```python
from build123d import *

# Parameters (mm, degrees)
CYLINDER004_R             = 1.65
CYLINDER004_DEPTH         = 15
CYLINDER004_ROLL_ANGLE    = -90
PAD004_DEPTH              = 2.5
FUSION006_PLACEMENT_ANGLE = 90
CYLINDER005_R             = 1.65
CYLINDER005_DEPTH         = 15
CYLINDER005_ROLL_ANGLE    = -90
PAD002_DEPTH              = 2.5
FUSION005_PLACEMENT_ANGLE = 90
PAD003_DEPTH              = 3
BOX009_W                  = 4
BOX009_H                  = 4
BOX009_DEPTH              = 10
BOX011_W                  = 24
BOX011_H                  = 12
BOX011_DEPTH              = 10
BOX010_W                  = 34
BOX010_H                  = 27
BOX010_DEPTH              = 3
FUSION007_PLACEMENT_ANGLE = -90


with BuildPart() as cylinder004:
    # Cylinder004 → Cylinder004 (new body)
    with BuildSketch(Plane.XY):
        Circle(CYLINDER004_R)
    extrude(amount=CYLINDER004_DEPTH)


with BuildPart() as cylinder004_1:
    # Cylinder004 roll: moved
    add(cylinder004.part.rotate(Axis((0, 0, 0), (1, 0, 0)), CYLINDER004_ROLL_ANGLE))


with BuildPart() as cylinder004_2:
    # Cylinder004 placement: moved
    add(cylinder004_1.part)


with BuildPart() as obj1:
    # Sketch → Pad004 (new body)
    with BuildSketch(Plane.XZ):
        Polygon((-3.348631, 0), (-1.674316, 2.9), (1.674316, 2.9), (3.348631, 0), (1.674316, -2.9), (-1.674316, -2.9), align=None)
    extrude(amount=PAD004_DEPTH)

    # Fusion006: union Cylinder004
    add(cylinder004_2.part)


with BuildPart() as obj1_1:
    # Fusion006 placement: moved
    add(obj1.part.moved(Location((1, -25, 28))).rotate(Axis((1, -25, 28), (0, 0, 1)), FUSION006_PLACEMENT_ANGLE))


with BuildPart() as cylinder005:
    # Cylinder005 → Cylinder005 (new body)
    with BuildSketch(Plane.XY):
        Circle(CYLINDER005_R)
    extrude(amount=CYLINDER005_DEPTH)


with BuildPart() as cylinder005_1:
    # Cylinder005 roll: moved
    add(cylinder005.part.rotate(Axis((0, 0, 0), (1, 0, 0)), CYLINDER005_ROLL_ANGLE))


with BuildPart() as cylinder005_2:
    # Cylinder005 placement: moved
    add(cylinder005_1.part)


with BuildPart() as obj2:
    # Sketch → Pad002 (new body)
    with BuildSketch(Plane.XZ):
        Polygon((-3.348631, 0), (-1.674316, 2.9), (1.674316, 2.9), (3.348631, 0), (1.674316, -2.9), (-1.674316, -2.9), align=None)
    extrude(amount=PAD002_DEPTH)

    # Fusion005: union Cylinder005
    add(cylinder005_2.part)


with BuildPart() as obj2_1:
    # Fusion005 placement: moved
    add(obj2.part.moved(Location((1, 25, 28))).rotate(Axis((1, 25, 28), (0, 0, 1)), FUSION005_PLACEMENT_ANGLE))


with BuildPart() as cut011:
    # Sketch001 → Pad003 (new body)
    with BuildSketch(Plane.YZ):
        with BuildLine():
            Line((-30, 14.925301), (30, 14.925301))
            Line((30, 27.925301), (30, 14.925301))
            ThreePointArc((30, 27.925301), (25, 32.925301), (20, 27.925301))
            ThreePointArc((13.035099, 19.925301), (18.35131, 22.328806), (20, 27.925301))
            Line((-13.035099, 19.925301), (13.035099, 19.925301))
            ThreePointArc((-20, 27.925301), (-18.35131, 22.328806), (-13.035099, 19.925301))
            ThreePointArc((-20, 27.925301), (-25, 32.925301), (-30, 27.925301))
            Line((-30, 27.925301), (-30, 14.925301))
        make_face()
    extrude(amount=PAD003_DEPTH)

    # Cut010: cut obj2
    add(obj2_1.part, mode=Mode.SUBTRACT)

    # Cut011: cut obj1
    add(obj1_1.part, mode=Mode.SUBTRACT)


with BuildPart() as cut011_1:
    # Cut011 placement: moved
    add(cut011.part.moved(Location((-17, -1.5, 0.374699))))


with BuildPart() as cubo009:
    # Box009 → Box009 (new body)
    with BuildSketch(Plane(origin=(10, -2, 10), x_dir=(1, 0, 0), z_dir=(0, 0, 1))):
        with Locations((2, 2)):
            Rectangle(BOX009_W, BOX009_H)
    extrude(amount=BOX009_DEPTH)


with BuildPart() as cubo011:
    # Box011 → Box011 (new body)
    with BuildSketch(Plane(origin=(-11.5, -6, 11), x_dir=(1, 0, 0), z_dir=(0, 0, 1))):
        with Locations((12, 6)):
            Rectangle(BOX011_W, BOX011_H)
    extrude(amount=BOX011_DEPTH)


with BuildPart() as obj3:
    # Box010 → Box010 (new body)
    with BuildSketch(Plane(origin=(-17, -13.5, 15), x_dir=(1, 0, 0), z_dir=(0, 0, 1))):
        with Locations((17, 13.5)):
            Rectangle(BOX010_W, BOX010_H)
    extrude(amount=BOX010_DEPTH)

    # Cut012: cut Cubo011
    add(cubo011.part, mode=Mode.SUBTRACT)

    # Cut009: cut Cubo009
    add(cubo009.part, mode=Mode.SUBTRACT)

    # Fusion007: union Cut011
    add(cut011_1.part)


with BuildPart() as obj3_1:
    # Fusion007 placement: moved
    add(obj3.part.moved(Location((0, 57, 0))).rotate(Axis((0, 57, 0), (0, 0, 1)), FUSION007_PLACEMENT_ANGLE))


solid = obj3_1.part
```
Part model, mm, in its own coordinate system. A direction names the side the tool comes from. Coordinates: 2 decimals unless noted, no trailing zeros. Write each loop counter-clockwise with the first axis right and the second up, starting at its lowest first coordinate (ties: lowest second). Pieces come first, ordered by that corner, then holes.
Item 1: Pin check, flat tips, straight feed: pin 1 (3.5 mm diameter, centred on y = 52.5, z = 17, fed in from +X); pin 2 (2 mm diameter, centred on x = -9, y = 60, fed in from +Z); pin 3 (2.5 mm diameter, centred on y = 54.5, z = 17, fed in from -X). Stop position of each tip, or through.
Item 2: Slice it at A-A (y = 62.5). Write the cut outline in (x, z), and give its area (3 significant figures).
Item 3: Slice it at C-C (z = 24.5). Write the cut outline in (x, y).
Item 4: Mould opens along Y. For faces 4 (the face through (-28, 73, 30)), 5 (the face through (-23, 73, 15.3)), 6 (the face through (-2, 44, 16)) say: released by +Y, released by -Y, zero draft, split by the parting line, or undercut.
Item 5: Slice it at D-D (x = -26.5). Write the cut outline in (y, z), and give its area (3 significant figures).
Item 6: Slice it at B-B (x = 0.5). Write the cut outline in (y, z).
Item 7: Which spindle directions (+Z, -Z, +X, -X, +Y, -Y) get a long thin tool onto all of the face, cutting with end or side? Do faces 1 (the face through (0, 68.5, 16)), 2 (the face through (20.977, 72.014, 29.804)), 3 (the face through (23.6, 72.5, 33.3)). Say none if no direction does.
Item 8: Probe line 1 (Y direction, x = 1, z = 17.5); line 2 (Z direction, x = 23.5, y = 73.35); line 3 (Y direction, x = -1.5, z = 20.25). List the from-to ranges inside material, lowest first.
Results found:
1. pin 1: stops at x = 13.5
1. pin 2: stops at z = 18
1. pin 3: stops at x = -13.5
2. outline: (-13.5, 15) - (-6, 15) - (-6, 18) - (-13.5, 18) - close; (6, 15) - (13.5, 15) - (13.5, 18) - (6, 18) - close
2. area: 45.0 mm2
3. outline: (-31.5, 71) - (-20.99, 71) - (-20.99, 74) - (-31.5, 74) - close; (17.99, 71) - (28.5, 71) - (28.5, 74) - (17.99, 74) - close
4. face 4: released by -Y
4. face 5: zero draft
4. face 6: undercut
5. outline: (71, 15.3) - (74, 15.3) - (74, 26.72) - (73, 26.72) - (73, 25.47) - (71, 25.47) - close; (71, 31.27) - (73, 31.27) - (73, 30.02) - (74, 30.02) - (74, 33.3) - (71, 33.3) - close
5. area: 39.1 mm2
6. outline: (40, 15) - (43, 15) - (43, 18) - (40, 18) - close; (68.5, 15) - (74, 15) - (74, 20.3) - (71, 20.3) - (71, 18) - (68.5, 18) - close
7. face 1: +Z, -Z
7. face 2: -Y
7. face 3: +Z, +Y, -Y
8. line 1: y = 40 to 43, 68.5 to 74
8. line 2: z = 15.3 to 26.72, 30.02 to 33.3
8. line 3: y = 71 to 74
